Input: dimensioned drawing with shaded views. Units: mm. Origin: part minimum x, y, z. A direction names the side the tool comes from. Coordinates: 2 decimals unless noted, no trailing zeros. Loops run counter-clockwise (first coordinate to the right, second up) from the corner with the lowest first, then second, coordinate; pieces in that order, holes last.
Item 1: Section query B-B, the plane x = 9. Return the cut outline in (y, z), then the cut area to 3 significant figures.
Item 2: Section query D-D, the plane y = 52.5. Return the cut outline in (x, z), then the cut area to 3 significant figures.
Item 3: Line query: probe 1 along X at (y, z) = (51.5, 55); probe 2 along X at (y, z) = (30, 55); probe 3 along Z at (x, y) = (54, 25). Output: solid intervals per line, ascending.
Item 4: Pin query (flat end, axial travel): pin 1 Ø6 at (y, z) = (7, 24) entering from -X; pin 2 Ø6 at (x, y) = (79, 12) entering from -Z; pin 3 Ø3.5 at (x, z) = (101, 55) entering from -Y; pin 4 Ø8 at (x, z) = (64, 98.5) entering from -Y. Return the tip coordinate at first contact, or that it passes through.
Item 5: Section query C-C, the plane x = 55. Return the cut outline in (y, z), then the cut area to 3 significant figures.
Item 6: Section query A-A, the plane z = 55. Return the cut outline in (x, y), then the cut area to 3 significant figures.
Item 7: Pull-direction query (Z, two-part tool) for the marked faces 4, 5 and 6; classes: +Z half, -Z half, draft (parallel to the pull), parting line (faces both ways), or undercut.
Item 8: Reachability of the marked faces 1, 2 and 3 from +Z, -Z, +X, -X, +Y, -Y: full face, straight path, thin tool, end or side. Return the list, or none.
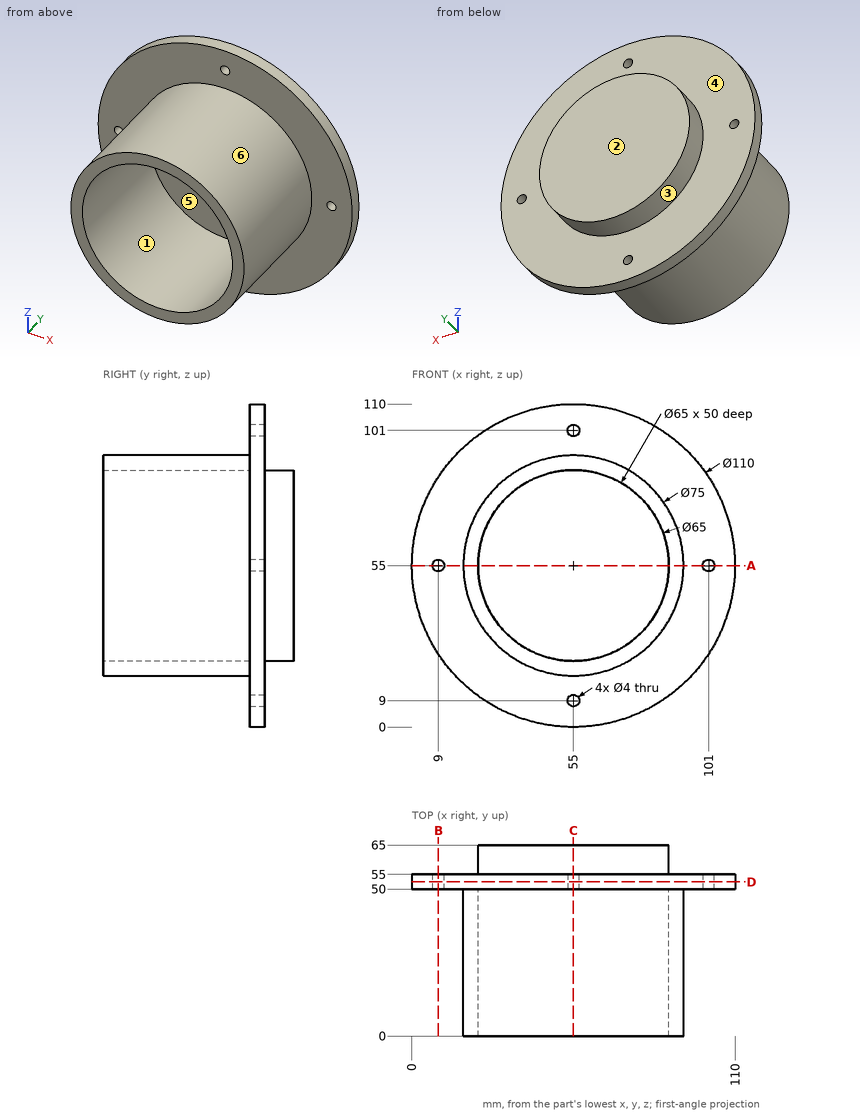
Verdict:
1. outline: (50, 24.85) - (55, 24.85) - (55, 53) - (50, 53) - close; (50, 57) - (55, 57) - (55, 85.15) - (50, 85.15) - close
1. area: 281 mm2
2. outline: circle Ø110 at (55, 55); hole circle Ø4 at (9, 55); hole circle Ø4 at (55, 9); hole circle Ø4 at (55, 101); hole circle Ø4 at (101, 55)
2. area: 9,450 mm2
3. probe 1: x = 0 to 7, 11 to 99, 103 to 110
3. probe 2: x = 17.5 to 22.5, 87.5 to 92.5
3. probe 3: z = 17.51 to 22.52, 87.48 to 92.49
4. pin 1: stops at x = 30.06
4. pin 2: stops at z = 23.93
4. pin 3: passes through
4. pin 4: stops at y = 50
5. outline: (0, 17.5) - (50, 17.5) - (50, 11) - (55, 11) - (55, 22.5) - (65, 22.5) - (65, 87.5) - (55, 87.5) - (55, 99) - (50, 99) - (50, 92.5) - (0, 92.5) - (0, 87.5) - (50, 87.5) - (50, 22.5) - (0, 22.5) - close; (50, 0) - (55, 0) - (55, 7) - (50, 7) - close; (50, 103) - (55, 103) - (55, 110) - (50, 110) - close
5. area: 1,660 mm2
6. outline: (0, 50) - (7, 50) - (7, 55) - (0, 55) - close; (11, 50) - (17.5, 50) - (17.5, 0) - (22.5, 0) - (22.5, 50) - (87.5, 50) - (87.5, 0) - (92.5, 0) - (92.5, 50) - (99, 50) - (99, 55) - (87.5, 55) - (87.5, 65) - (22.5, 65) - (22.5, 55) - (11, 55) - close; (103, 50) - (110, 50) - (110, 55) - (103, 55) - close
6. area: 1,660 mm2
7. face 4: draft
7. face 5: undercut
7. face 6: parting line
8. face 1: -Y
8. face 2: +Z, -Z, +X, -X, +Y
8. face 3: +Y
